from build123d import *

# Parameters (mm, degrees)
F0_W     = 2.54
F0_H     = 2.54
F1_DEPTH = 2.54
F2_W     = 1.397
F2_H     = 35.56
F3_DEPTH = 2.541
F4_W     = 3.81
F4_H     = 3.81
F5_DEPTH = 2.541


with BuildPart() as f1:
    # F0 (on Top) → F1 (new body)
    with BuildSketch(Plane.XY):
        Polygon((6.35, 25.4), (-6.35, 25.4), (-6.35, -12.7), (-1.27, -12.7), (1.27, -12.7), (6.35, -12.7), align=None)
        with Locations((0, -13.97)):
            Rectangle(F0_W, F0_H)
        Polygon((1.27, -15.24), (-1.27, -15.24), (-3.302, -15.24), (-3.302, -21.59), (3.048, -21.59), (3.048, -15.24), align=None)
    extrude(amount=F1_DEPTH)

    # F2 (on face) → F3 (cut, through all)
    with BuildSketch(Plane.XY.offset(2.54)):
        with Locations((-4.2545, 6.35)):
            Rectangle(F2_W, F2_H)
        with Locations((-1.4605, 6.35)):
            Rectangle(F2_W, F2_H)
        with Locations((1.3335, 6.35)):
            Rectangle(F2_W, F2_H)
        with Locations((4.1275, 6.35)):
            Rectangle(F2_W, F2_H)
    extrude(amount=-F3_DEPTH, mode=Mode.SUBTRACT)

    # F4 (on face) → F5 (cut, through all)
    with BuildSketch(Plane.XY.offset(2.54)):
        with Locations((-0.127, -18.415)):
            Rectangle(F4_W, F4_H)
    extrude(amount=-F5_DEPTH, mode=Mode.SUBTRACT)


solid = f1.part
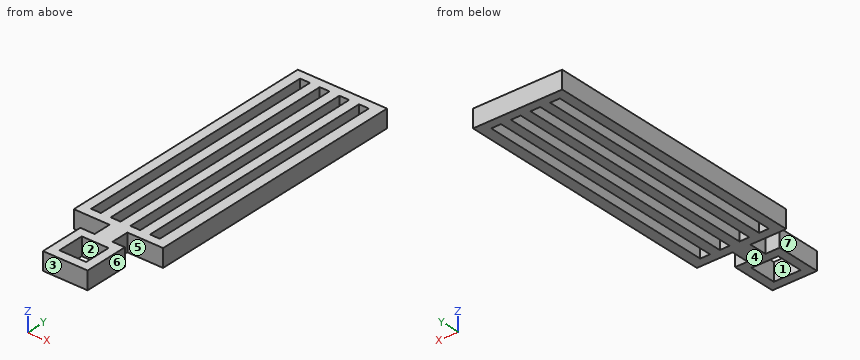
Can you work these out from the model? Positions are in its coordinate system, mm. Face numbers are marked on the shaded views. A direction names the side the tool comes from. Round coordinates to 2 decimals unless told otherwise and drop trailing zeros. Loops run counter-clockwise (first coordinate to the right, second up) from the corner with the lowest first, then second, coordinate; pieces in that order, holes last. Notation, with made-up numbers: (87.5, 49) - (104.5, 49) arc R28 ccw to (104.5, 82) - close; hole circle Ø5 at (57.25, 18.25). An arc over 180 degrees is marked (long way). Answer in a Markdown table with one row per item. Add a question column.
Q1. I need wall thicknesses on L1, parallel to X at y = 1, z = 2.35 (3 decimals); L2, parallel to Y at x = 1.5, z = 1.3; L3, parallel to Y at x = -2.25, z = 1.3. Which ranges of each line are inside material? Lowest first, please.
Q2. I want a section at C-C on z = 1.55. Count the separate pieces of the cut face and the enclosed holes in it, and give its area (3 significant figures).
Q3. I want a section at B-B on y = 13. List the corners of the cut face in (x, z) for me (3 decimals), and give its area (3 significant figures).
Q4. I want a section at A-A on x = -0.25. List the corners of the cut face in (y, z) for me, and give its area (3 significant figures).
Q5. Which directions (+Z, -Z, +X, -X, +Y, -Y) give clear straight access to the entire face, cutting with the end or side of a thin tool? Please do the marked faces 5, 6 and 7.
Q6. I want a section at D-D on x = -4.5. List the corners of the cut face in (y, z) for me, and give its area (3 significant figures).
Q7. We'd pull the mould along Y, two halves only. Please class the marked faces 1, 2, 3 and 4: pulls with the +Y half, pulls with the -Y half, needs draft (parallel to the pull), parting line crosses it, or undercut.
Q8. For pin 1 Ø1.5 at (x, z) = (4, 1.5) entering from -Y; pin 2 Ø0.8 at (y, z) = (-18.5, 1.5) entering from -X; pin 3 Ø1.3 at (y, z) = (-14.5, 1.5) entering from -X, each with a flat end and sliding along its axis, tell me the tip position at first contact or that it passes through.
A:
| question | item | result |
|---|---|---|
| 1 | L1 | -6.35 to -4.953, -3.556 to -2.159, -0.762 to 0.635, 2.032 to 3.429, 4.826 to 6.35 |
| 1 | L2 | -21.59 to -20.32, -16.51 to -15.24, -12.7 to -11.43, 24.13 to 25.4 |
| 1 | L3 | -21.59 to -15.24, -12.7 to 25.4 |
| 2 | separate pieces | 1 |
| 2 | enclosed holes | 5 |
| 2 | area | 317 mm^2 |
| 3 | outline | (-6.35, 0) - (-4.953, 0) - (-4.953, 2.54) - (-6.35, 2.54) - close; (-3.556, 0) - (-2.159, 0) - (-2.159, 2.54) - (-3.556, 2.54) - close; (-0.762, 0) - (0.635, 0) - (0.635, 2.54) - (-0.762, 2.54) - close; (2.032, 0) - (3.429, 0) - (3.429, 2.54) - (2.032, 2.54) - close; (4.826, 0) - (6.35, 0) - (6.35, 2.54) - (4.826, 2.54) - close |
| 3 | area | 18.1 mm^2 |
| 4 | outline | (-21.59, 0) - (-20.32, 0) - (-20.32, 2.54) - (-21.59, 2.54) - close; (-16.51, 0) - (25.4, 0) - (25.4, 2.54) - (-16.51, 2.54) - close |
| 4 | area | 110 mm^2 |
| 5 | face 5 | +Z, -Z, +X |
| 5 | face 6 | +Z, -Z, +X, -Y |
| 5 | face 7 | +Z, -Z, -X, -Y |
| 6 | outline | (-12.7, 0) - (-11.43, 0) - (-11.43, 2.54) - (-12.7, 2.54) - close; (24.13, 0) - (25.4, 0) - (25.4, 2.54) - (24.13, 2.54) - close |
| 6 | area | 6.45 mm^2 |
| 7 | face 1 | undercut |
| 7 | face 2 | undercut |
| 7 | face 3 | pulls with the -Y half |
| 7 | face 4 | needs draft |
| 8 | pin 1 | y = -12.7 |
| 8 | pin 2 | x = -3.3 |
| 8 | pin 3 | x = -1.27 |
